Could you check a few things on this model? Use its own coordinates, in mm. Give positions to 0.01 mm unless a question says otherwise; leave off trailing zeros. Order: outer loops, then holes, each group sorted by start corner. A loop starts at its lowest first (then second) coordinate and runs counter-clockwise, first axis right, second up.
from build123d import *

# Parameters (mm, degrees)
SKETCH_1_W             = 160
SKETCH_1_H             = 220
SM_BASE_FLANGE_1_DEPTH = 16
SKETCH_2_R             = 11.5
CUT_EXTRUDE_1_DEPTH    = 30


# Sheet-metal steps are written as plain solids
with BuildPart() as part:
    # Sketch 1 → Базовая кромка1 (new body)
    with BuildSketch(Plane.XY):
        with Locations((80, -110)):
            Rectangle(SKETCH_1_W, SKETCH_1_H)
    extrude(amount=-SM_BASE_FLANGE_1_DEPTH)

    # Sketch 2 → Вырез-Вытянуть1 (cut)
    with BuildSketch(Plane(origin=(0, 0, -16), x_dir=(-1, 0, 0), z_dir=(0, 0, -1))):
        with Locations((-30, -165)):
            Circle(SKETCH_2_R)
        with Locations((-30, -65)):
            Circle(SKETCH_2_R)
        with Locations(Location((-130, -165, 0), (0, 0, 180))):
            Circle(SKETCH_2_R)
        with Locations(Location((-130, -65, 0), (0, 0, 180))):
            Circle(SKETCH_2_R)
    extrude(amount=-CUT_EXTRUDE_1_DEPTH, mode=Mode.SUBTRACT)


solid = part.part
Item 1: Please list where these lines run through material, in increasing order: line 1 along Y through (x, z) = (130, -6.75); line 2 along X through (y, z) = (-159, -12); line 3 along Y through (x, z) = (138.5, -8.25).
Findings:
line 1: y = -220 to -176.5, -153.5 to -76.5, -53.5 to 0
line 2: x = 0 to 20.19, 39.81 to 120.19, 139.81 to 160
line 3: y = -220 to -172.75, -157.25 to -72.75, -57.25 to 0
Item 2: Imagine slicing it at B-B on x = 130. List the corners of the cut face in (y, z) for me, then the cut area to 3 significant figures.
Findings:
outline: (-220, -16) - (-176.5, -16) - (-176.5, 0) - (-220, 0) - close; (-153.5, -16) - (-76.5, -16) - (-76.5, 0) - (-153.5, 0) - close; (-53.5, -16) - (0, -16) - (0, 0) - (-53.5, 0) - close
area: 2,780 mm2
Item 3: Imagine slicing it at C-C on y = -165. List the corners of the cut face in (x, z) for me.
Findings:
outline: (0, -16) - (18.5, -16) - (18.5, 0) - (0, 0) - close; (41.5, -16) - (118.5, -16) - (118.5, 0) - (41.5, 0) - close; (141.5, -16) - (160, -16) - (160, 0) - (141.5, 0) - close
Item 4: Imagine slicing it at A-A on z = -11. List the corners of the cut face in (x, y) for me.
Findings:
outline: (0, -220) - (160, -220) - (160, 0) - (0, 0) - close; hole circle Ø23 at (30, -165); hole circle Ø23 at (30, -65); hole circle Ø23 at (130, -165); hole circle Ø23 at (130, -65)
